```python
from build123d import *

# Parameters (mm, degrees)
BOSS_EXTRUDE1_DEPTH = 25.4
CHAMFER1_SIZE       = 15
CHAMFER1_SIZE_2     = 25.980762114


with BuildPart() as part:
    # Sketch1 → Boss-Extrude1 (new body)
    with BuildSketch(Plane(origin=(0, 0, 0), x_dir=(1, 0, 0), z_dir=(0, 1, 0))):
        with BuildLine():
            ThreePointArc((-10, -8.415), (0, 1.585), (10, -8.415))
            Line((10, -8.415), (10, -15.463254024))
            ThreePointArc((10, -15.463254024), (16.17501507, -8.802335628), (18.415, 0))
            ThreePointArc((18.415, 0), (-8.802335628, 16.17501507), (-10, -15.463254024))
            Line((-10, -15.463254024), (-10, -8.415))
        make_face()
    extrude(amount=BOSS_EXTRUDE1_DEPTH)

    # Chamfer1
    # the kernel refuses this chamfer: 25.980762114, 15 mm, written as the material it takes off along each edge
    with BuildSketch(Plane(origin=(0, 25.4, 8.415), x_dir=(-1, 0, 0), z_dir=(0, 0, 1))) as chamfer1_piece_1:
        Polygon((10 + CHAMFER1_SIZE, 0), (10, CHAMFER1_SIZE_2), (10, 0), align=None)
    revolve(axis=Axis((0, 25.4, 8.415), (0, -1, 0)), revolution_arc=180, mode=Mode.SUBTRACT)
    with BuildSketch(Plane(origin=(-10, 25.4, 82.677713582), x_dir=(0.019326765612700622, -0.9998132206222078, 0), z_dir=(0, 0, -1))) as chamfer1_piece_2:
        Polygon((CHAMFER1_SIZE_2 * 0.999813220604, CHAMFER1_SIZE_2 * 0.0193267656124), (-CHAMFER1_SIZE * 0.0193267656127, CHAMFER1_SIZE * 0.999813220622), (0, 0), align=None)
    extrude(amount=74.262713582, mode=Mode.SUBTRACT)
    with BuildSketch(Plane(origin=(10, 25.4, 8.415), x_dir=(0.9983227437537926, 0.05789386240267136, 0), z_dir=(0, 0, 1))) as chamfer1_piece_3:
        Polygon((CHAMFER1_SIZE * 0.998322743754, -CHAMFER1_SIZE * 0.0578938624027), (-CHAMFER1_SIZE_2 * 0.0578938624016, -CHAMFER1_SIZE_2 * 0.998322743736), (0, 0), align=None)
    extrude(amount=74.262713582, mode=Mode.SUBTRACT)


solid = part.part
```
Read the model definition and answer for the solid it produces. Units are mm, in the model's axes. A direction names the side the tool comes from. Give positions to 0.01 mm unless a question says otherwise; leave off trailing zeros. Write each loop counter-clockwise with the first axis right and the second up, starting at its lowest first coordinate (ties: lowest second). Pieces come first, ordered by that corner, then holes. Notation, with made-up numbers: (-1.5, 17.25) - (46.5, 17.25) arc R19 cw to (46.5, 34.25) - close; hole circle Ø3 at (86.25, 69). An arc over 180 degrees is marked (long way). Write item = value, one per line. Start each with the question number.
Item 1: Find section C-C (x = 0). Give the vertices of the cut face in (y, z) (3 decimals), then the cut area to 3 significant figures.
Item 2: Find section B-B (y = 3.5). Give the vertices of the cut face in (x, z) (3 decimals).
Item 3: Find the intervals of material crossed by probe 1 along X at (y, z) = (14.25, 2); probe 2 along Y at (x, z) = (-12.5, 11.5); probe 3 along Z at (x, y) = (14.5, 18), in increasing order. Write a range as [from, to].
Item 4: Find section D-D (y = 7.5). Give the vertices of the cut face in (x, z) (3 decimals), then the cut area to 3 significant figures.
Item 5: Each of these flat-tipped pins is pushed along its axis until it touches: P1, Ø2, axis at y = 9, z = -14, coming from the -X side; P2, Ø5, axis at x = -10, y = 11.5, coming from the -Z side; P3, Ø5, axis at x = -3, y = 8, coming from the +Z side; P4, Ø10, axis at x = 14.5, z = -9, coming from the +Y side. Where does it stop, or does it pass through?
Item 6: Find section A-A (z = 13.5). Give the vertices of the cut face in (x, y).
Item 7: A tool of negligible diameter and unlimited length cuts with its end or side. For faces 1 (the flat face through (0, 25.4, -17)), 2 (the flat face through (12.728, 4.145, 11.022)), from which of +Z, -Z, +X, -X, +Y, -Y can it reach the whole face along a straight path? Write none if from no direction.
Response:
q1.outline = (0, -18.415) - (25.4, -18.415) - (25.4, -16.585) - (0, -1.92) - close
q1.area = 233 mm²
q2.outline = (-12.356, 8.415) - (-12.356, 13.654) arc R18.415 ccw (long way) to (12.356, 13.654) - (12.356, 8.415) arc R12.356 cw to start
q3.probe_1 = [-18.31, -17.42], [17.42, 18.31]
q3.probe_2 = [0, 3.75]
q3.probe_3 = [-11.35, -6.4]
q4.outline = (-14.665, 8.415) - (-14.665, 11.137) arc R18.415 ccw (long way) to (14.665, 11.137) - (14.665, 8.415) arc R14.665 cw to start
q4.area = 499 mm²
q5.P1 = -13.04
q5.P2 = -16.82
q5.P3 = -4.61
q5.P4 = 25.4
q6.outline = (-12.52, 0) - (-10.34, 0) - (-12.52, 3.79) - close; (10.34, 0) - (12.52, 0) - (12.52, 3.79) - close
q7.face_1 = +Z, -Z, +X, -X, +Y
q7.face_2 = +Z, +Y
